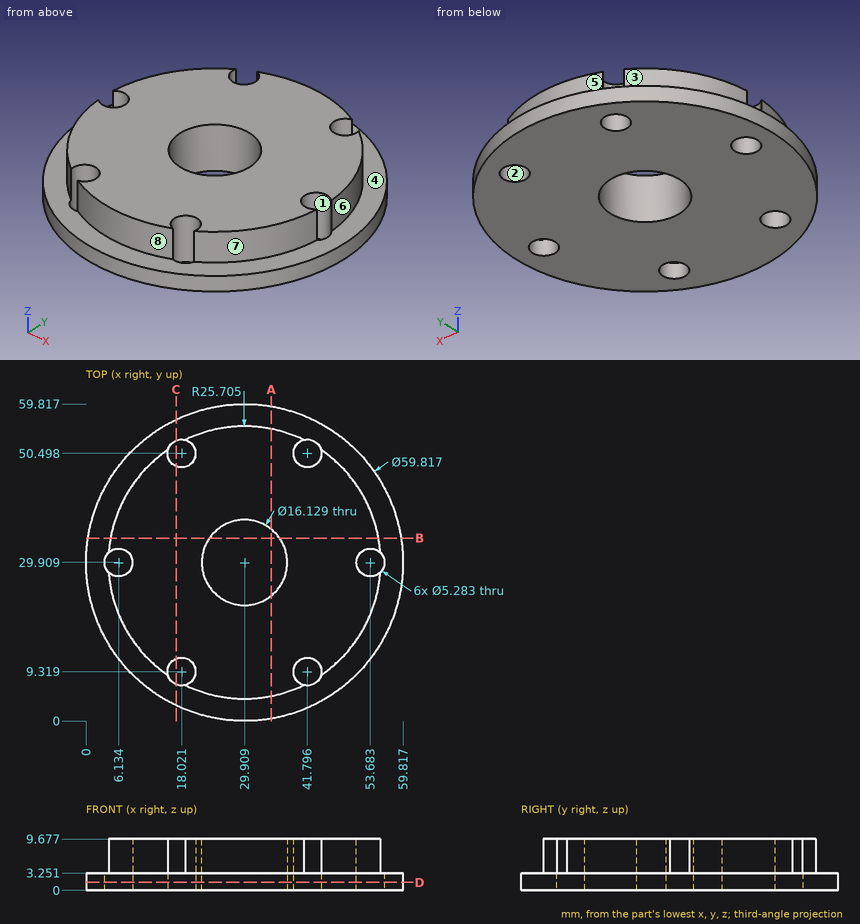
The drawing under review shows one solid part. Ordinate dimensions are in mm from its lowest x, y, z. A direction names the side the tool comes from. Give positions to 0.01 mm unless a question says otherwise; leave off trailing zeros. Order: outer loops, then holes, each group sorted by start corner. A loop starts at its lowest first (then second) coordinate and runs counter-clockwise, first axis right, second up. Notation, with made-up numbers: M 43,4.25 L 88,4.25 A18 cw 88,9.25 Z; hole C 9.25,56.5 d2. An arc over 180 degrees is marked long. One line per question, with ' | ' between items. Start each with the question number.
Q1. We need section C-C (x = 17). Write out the cut boundary in (y, z) (1 decimal).
Q2. The part is to be moulded in two halves that separate along Y. For the marked faces 1, 2, 3 and 4, say which applies: +Y half, -Y half, draft (parallel to the pull), parting line (faces both ways), or undercut.
Q3. We need section B-B (y = 34.5). Write out the cut boundary in (x, z) (1 decimal).
Q4. For pin 1 Ø2 at (x, y) = (20, 20.5) entering from -Z; pin 2 Ø1.5 at (x, z) = (38, 4.5) entering from +Y; pin 3 Ø1 at (x, z) = (40.5, 2) entering from +Y; pin 4 Ø2 at (x, z) = (49.5, 5) entering from +Y, all flat-tipped, find the tip position at first contact; note any pin that passes through.
Q5. We need section A-A (x = 35). Write out the cut boundary in (y, z) (1 decimal).
Q6. For L1, parallel to Y at x = 40.5, z = 7.5 (1 decimal); L2, parallel to X at y = 11, z = 4 (1 decimal); L3, parallel to X at y = 49, z = 6.5 (1 decimal), list the stretches that pass through material, from the lowest coordinate up. Write a range as [from, to].
Q7. We need section D-D (z = 1.5). Write out the cut boundary in (x, y) (1 decimal), plus the area to 3 significant figures.
Q8. Machinability: for the marked faces 5, 6, 7 and 8, which of the approach directions +Z, -Z, +X, -X, +Y, -Y give a long, thin tool a straight path to every point of the face, cutting with its end or side? Answer none if there is none.
Returned:
1) outline: M 2.9,0 L 6.9,0 L 6.9,3.3 L 2.9,3.3 Z; M 11.8,0 L 48.1,0 L 48.1,9.7 L 11.8,9.7 Z; M 52.9,0 L 56.9,0 L 56.9,3.3 L 52.9,3.3 Z
2) face 1: undercut | face 2: undercut | face 3: +Y half | face 4: draft
3) outline: M 0.4,0 L 23.3,0 L 23.3,9.7 L 4.6,9.7 L 4.6,3.3 L 0.4,3.3 Z; M 36.5,0 L 59.5,0 L 59.5,3.3 L 55.2,3.3 L 55.2,9.7 L 36.5,9.7 Z
4) pin 1: z = 0 | pin 2: y = 54.54 | pin 3: y = 58.06 | pin 4: y = 47.66
5) outline: M 0.4,0 L 23.7,0 L 23.7,9.7 L 4.7,9.7 L 4.7,3.3 L 0.4,3.3 Z; M 36.2,0 L 59.4,0 L 59.4,3.3 L 55.1,3.3 L 55.1,9.7 L 36.2,9.7 Z
6) L1: [6.5, 7], [11.6, 48.2], [52.8, 53.3] | L2: [12.5, 16], [20.1, 39.8], [43.8, 47.3] | L3: [12.7, 15.8], [20.2, 39.6], [44, 47.1]
7) outline: C 29.9,29.9 d59.8; hole C 6.1,29.9 d5.3; hole C 18,9.3 d5.3; hole C 18,50.5 d5.3; hole C 29.9,29.9 d16.1; hole C 41.8,9.3 d5.3; hole C 41.8,50.5 d5.3; hole C 53.7,29.9 d5.3 | area: 2,470 mm2
8) face 5: +Z, +Y | face 6: +Z, +X, +Y | face 7: +Z, +X, -Y | face 8: +Z, -Y
